Autodesk Fusion 360 part; units mm, degrees
sketch "Sketch1" plane through (0, 0, 0) normal (0, 0, 1) x (1, 0, 0)
  line L0 (0, 0) -> (200, 0)
  line L1 (200, 0) -> (200, 200)
  line L2 (200, 200) -> (0, 200)
  line L3 (0, 200) -> (0, 0)
  dimension "d1" = 200
  dimension "d2" = 200
extrude "Extrude1" add sketch "Sketch1" along normal blind 12 makes body 1
sketch "Sketch2" plane through (0, 0, 0) normal (0, 0, 1) x (1, 0, 0)
  circle A0 centre (50, 40) radius 38.95
  circle A1 centre (50, 40) radius 39.575
  circle A2 centre (50, 40) radius 39.325
  dimension "d5" = 77.9
  dimension "d6" = 79.15
  dimension "d15" = 78.65
extrude "Extrude2" add sketch "Sketch2" along normal blind 0.1 separate body contours A0 | A1 | A2 makes body 2
extrude "Extrude3" cut sketch "Sketch2" along normal blind 2.55 contours A1 | A2 bodies 2
extrude "Extrude5" add sketch "Sketch2" along normal blind 3.8 contours A1 | A2 bodies 2
extrude "Extrude4" cut sketch "Sketch2" along normal blind 2.55 contours A2 bodies 2 makes body 3 at (55.9532, 44.0588, 0)
extrude "Extrude6" add sketch "Sketch2" along normal blind 0.1 contours A2 bodies 2 3
extrude "Extrude7" add sketch "Sketch2" along normal blind 3 separate body contours A2 makes body 4
move_body "Move1" bodies 4 to x (1, 0, 0) y (0, 1, 0) z (0, 0, 1) at (0, 0, 3.55)
combine "Combine1" operation cut target body 2 tool bodies 4
extrude "Extrude8" cut 1 faces at (88.1759, 49.7182, 3.8) along direction (0, 0, -1) blind 0.24 on bodies 2 bodies 2
extrude "Extrude9" add 1 faces at (88.1759, 49.7182, 3.56) along direction (0, 0, 1) blind 1.5 on bodies 2 bodies 2
copy_body "CopyPasteBodies1" bodies 1 makes body 5
extrude "Extrude10" cut sketch "Sketch2" along normal blind 25 contours A0 | A1 | A2 keep common part bodies 5
extrude "Extrude11" add sketch "Sketch2" along normal blind 20 separate body contours A1 | A2 makes body 6
move_body "Move2" bodies 6 to x (1, 0, 0) y (0, 1, 0) z (0, 0, 1) at (0, 0, 1.8)
combine "Combine2" operation cut target body 5 tool bodies 6
draft "Draft2" angle -4 neutral plane through (0, 0, 0) pull (0, 0, -1) 1 faces at (88.7564, 43.8782, 8.6) on bodies 5
sketch "AirHole" plane through (0, 0, 0) normal (0, 0, 1) x (1, 0, 0)
  circle A0 centre (50, 40) radius 3
  circle A1 centre (50, 40) radius 0.5
  dimension "d28" = 6
  dimension "d29" = 1
extrude "Extrude12" cut sketch "AirHole" along normal blind 26 contours A0 | A1 bodies 5
sketch "Sketch4" plane through (0, 0, 0) normal (0, 0, 1) x (1, 0, 0)
  circle A0 centre (50, 40) radius 42.1814
extrude "Extrude13" add sketch "Sketch4" along normal blind 1 bodies 5
extrude "Extrude14" cut sketch "AirHole" along normal blind 15 contours A0 | A1 bodies 5
sketch "Sketch5" plane through (0, 0, 0) normal (1, 0, 0) x (0, 1, 0)
sketch "Sketch6" plane through (0, 0, 0) normal (1, 0, 0) x (0, 1, 0)
sketch "Sketch7" plane through (0, 0, 0) normal (0, 0, 1) x (1, 0, 0)
  circle A0 centre (50, 40) radius 42.2
  circle A1 centre (50, 40) radius 42.2
  circle A2 centre (50, 40) radius 48.2
  circle A3 centre (50, 40) radius 55.2268
  dimension "d41" = 84.4
  dimension "d42" = 96.4
extrude "Extrude15" add sketch "Sketch7" along normal blind 12 separate body contours A3 makes body 7
hidden bodies 1 2 7
equation "d3 = WoodHeight"
equation "d5 = d6 - 1.25 mm"
equation "d15 = d6 - 0.5 mm"
equation "WoodHeight = 12 mm"
equation "d42 = d41 + 12 mm"
equation "CutDim = 6 mm"
equation "d44 = WoodHeight"
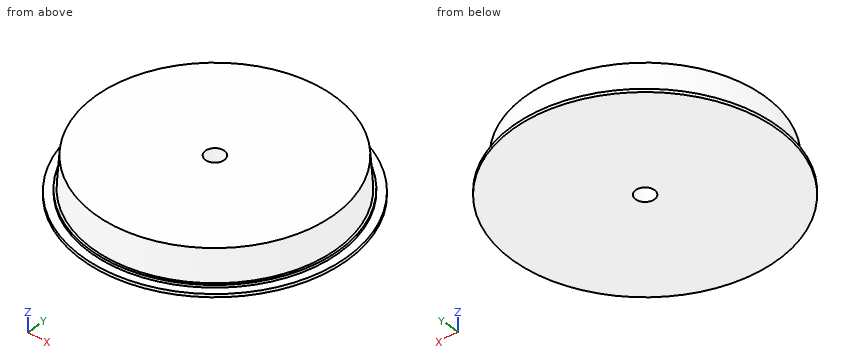
Input: part model. Units: mm. Frame: model coordinates. Coordinates: 2 decimals unless noted, no trailing zeros. Order: outer loops, then holes, each group sorted by start corner. A loop starts at its lowest first (then second) coordinate and runs counter-clockwise, first axis right, second up. Notation, with made-up numbers: M 36,29.25 L 50,29.25 A23 cw 50,49.25 Z; hole C 55.25,17 d9. An arc over 180 degrees is marked long. One line per question, with ' | ' between items.
Item 1: Ray query, line 1 along Y through (x, z) = (50, 6.25); line 2 along Z through (x, y) = (21, 11.5); line 3 along Y through (x, z) = (50, 3.5). Return the intervals inside material, ascending.
Geometry results:
line 1: y = 1.49 to 37, 43 to 78.51 | line 2: z = 0 to 1 | line 3: y = 1.29 to 37, 43 to 78.71
Item 2: Section B-B (y = 40). Output: boundary loops of the cut face in (x, z) (3 decimals).
Geometry results:
outline: M 7.819,0 L 47,0 L 47,12 L 11.889,12 L 11.176,1.8 L 10.425,1.8 L 10.425,1 L 7.819,1 Z; M 53,0 L 92.181,0 L 92.181,1 L 89.575,1 L 89.575,1.8 L 88.824,1.8 L 88.111,12 L 53,12 Z
Item 3: Section A-A (x = 50). Output: boundary loops of the cut face in (y, z) (3 decimals).
Geometry results:
outline: M -2.181,0 L 37,0 L 37,12 L 1.889,12 L 1.176,1.8 L 0.425,1.8 L 0.425,1 L -2.181,1 Z; M 43,0 L 82.181,0 L 82.181,1 L 79.575,1 L 79.575,1.8 L 78.824,1.8 L 78.111,12 L 43,12 Z
Item 4: Pin query (flat end, axial travel): pin 1 (3 mm diameter, centred on x = 82.5, z = 10, fed in from -Y); pin 2 (1 mm diameter, centred on x = 73, z = 2.5, fed in from -Y); pin 3 (5 mm diameter, centred on y = 58.5, z = 3, fed in from -X). Return the tip coordinate at first contact, or that it passes through.
Geometry results:
pin 1: stops at y = 17.58 | pin 2: stops at y = 8.42 | pin 3: stops at x = 11.4
Item 5: Section C-C (z = 7). Output: boundary loops of the cut face in (x, y).
Geometry results:
outline: C 50,40 d76.92; hole C 50,40 d6
